Part print with two shaded views. Sizes in mm from the minimum x, y, z corner. A direction names the side the tool comes from. Round coordinates to 2 decimals unless told otherwise and drop trailing zeros. Loops run counter-clockwise (first coordinate to the right, second up) from the corner with the lowest first, then second, coordinate; pieces in that order, holes last.
(1) Tool access for the marked faces 4, 5, 6, 7 and 8: list every direction of +Z, -Z, +X, -X, +Y, -Y with a clear straight run to the whole face (end or side of a thin tool).
(2) Flat gauge pins, fed straight in: pin 1 (8 mm diameter, centred on x = 26.5, z = 11.5, fed in from +Y); pin 2 (2 mm diameter, centred on x = 12, y = 2.5, fed in from -Z); pin 3 (1.6 mm diameter, centred on x = 12, y = 2.5, fed in from +Z); pin 4 (0.9 mm diameter, centred on x = 35, z = 12.5, fed in from +Y). Where does each tip first touch, or does it go through?
(3) Mould opens along X. For the marked faces 1, 2 and 3 say: +X half, -X half, draft (parallel to the pull), parting line (faces both ways), or undercut.
(4) Probe probe 1 along X at (y, z) = (0.65, 12.5); probe 2 along X at (y, z) = (2.8, 3); probe 3 along X at (y, z) = (3.9, 9.5). List the from-to ranges inside material, lowest first.
(5) Cut at A-A on y = 2.4. List the corners of the cut face in (x, z), then the cut area to 3 significant figures.
(6) Cut at C-C on y = 4.35. List the corners of the cut face in (x, z), then the cut area to 3 significant figures.
(7) Cut at D-D on z = 4.5. List the corners of the cut face in (x, y), then the cut area to 3 significant figures.
(8) Cut at B-B on x = 2. List the corners of the cut face in (y, z), then the cut area to 3 significant figures.
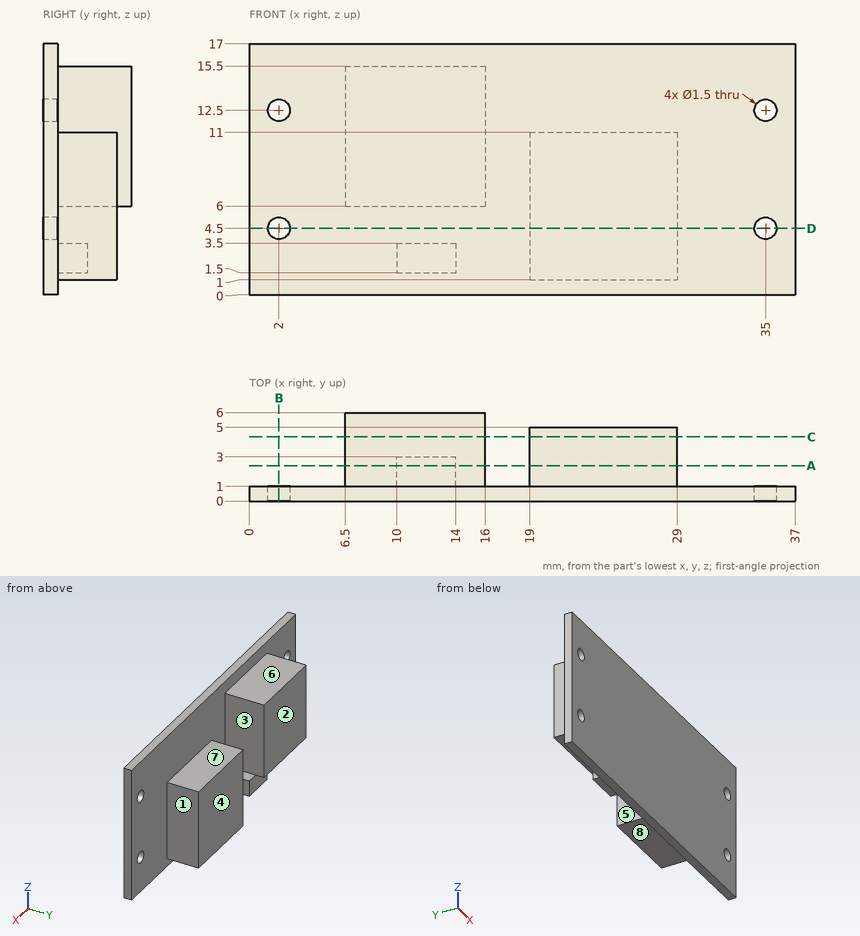
Final values:
1. face 4: +Z, -Z, +X, +Y
1. face 5: +Z, -Z, +Y
1. face 6: +Z, +X, -X, +Y
1. face 7: +Z, +X, +Y
1. face 8: -Z, +X, -X, +Y
2. pin 1: stops at y = 5
2. pin 2: stops at z = 1.5
2. pin 3: stops at z = 15.5
2. pin 4: passes through
3. face 1: +X half
3. face 2: draft
3. face 3: undercut
4. probe 1: x = 0 to 1.25, 2.75 to 34.25, 35.75 to 37
4. probe 2: x = 10 to 14, 19 to 29
4. probe 3: x = 6.5 to 16, 19 to 29
5. outline: (6.5, 6) - (16, 6) - (16, 15.5) - (6.5, 15.5) - close; (10, 1.5) - (14, 1.5) - (14, 3.5) - (10, 3.5) - close; (19, 1) - (29, 1) - (29, 11) - (19, 11) - close
5. area: 198 mm2
6. outline: (6.5, 6) - (16, 6) - (16, 15.5) - (6.5, 15.5) - close; (19, 1) - (29, 1) - (29, 11) - (19, 11) - close
6. area: 190 mm2
7. outline: (0, 0) - (1.25, 0) - (1.25, 1) - (0, 1) - close; (2.75, 0) - (34.25, 0) - (34.25, 1) - (29, 1) - (29, 5) - (19, 5) - (19, 1) - (2.75, 1) - close; (35.75, 0) - (37, 0) - (37, 1) - (35.75, 1) - close
7. area: 74.0 mm2
8. outline: (0, 0) - (1, 0) - (1, 3.75) - (0, 3.75) - close; (0, 5.25) - (1, 5.25) - (1, 11.75) - (0, 11.75) - close; (0, 13.25) - (1, 13.25) - (1, 17) - (0, 17) - close
8. area: 14.0 mm2
